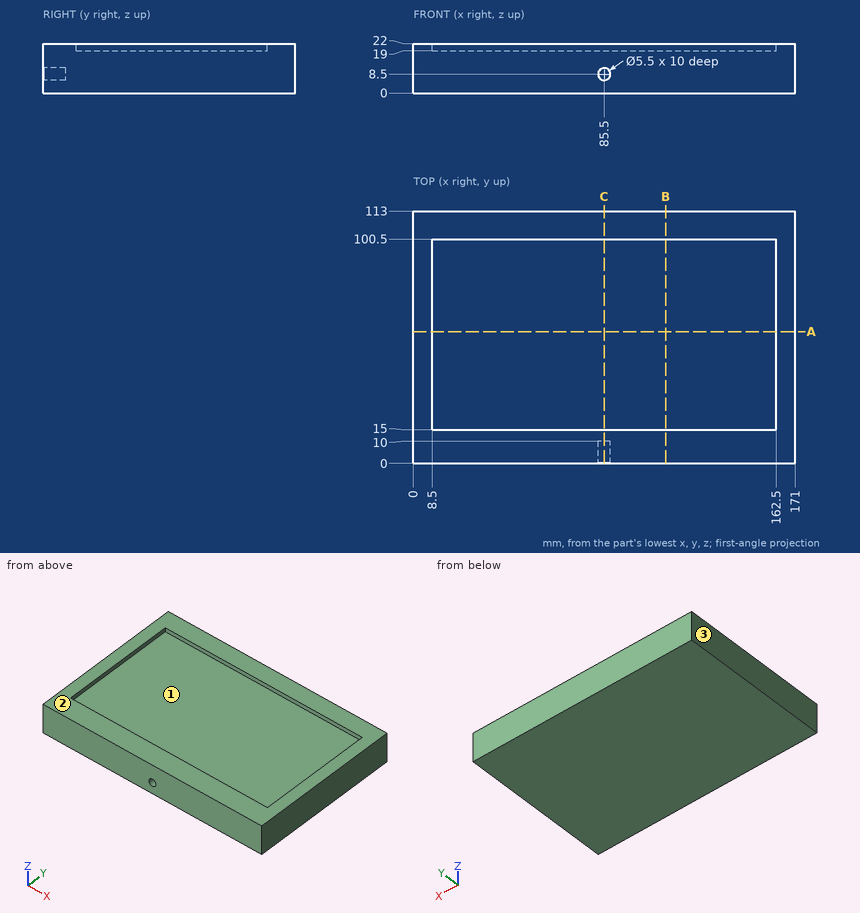
Input: dimensioned drawing with shaded views. Units: mm. Origin: part minimum x, y, z. Give positions to 0.01 mm unless a question says otherwise; leave off trailing zeros. Write each loop counter-clockwise with the first axis right and the second up, starting at its lowest first coordinate (ties: lowest second). Pieces come first, ordered by that corner, then holes. Notation, with made-up numbers: (-32.75, -12) - (-11.75, -12) arc R8 cw to (-11.75, -7) - close; hole circle Ø8 at (49.5, 59.5). An arc over 180 degrees is marked (long way). One line per item, written item: value. Start each with the question number.
Q1. Section query C-C, the plane x = 85.5. Return the cut outline in (y, z), then the cut area to 3 significant figures.
Q2. Draft query along X for the marked faces 1, 2 and 3. Return one class per face: +X half, -X half, draft (parallel to the pull), parting line (faces both ways), or undercut.
Q3. Material intervals for probe 1 along Z at (x, y) = (85.5, 2.75); probe 2 along Y at (x, z) = (102, 21); probe 3 along X at (y, z) = (27.5, 20.5), sorted ascending. Write a range as from..to.
Q4. First-contact query: pin 1 Ø1.6 at (x, z) = (85, 8) entering from -Y; pin 2 Ø10 at (x, y) = (142, 87) entering from +Z; pin 3 Ø8 at (x, y) = (145, 65.5) entering from -Z. Flat tips, straight axial feed; report the tip coordinate or a pass-through.
Q5. Section query B-B, the plane x = 113. Return the cut outline in (y, z), then the cut area to 3 significant figures.
Q6. Section query A-A, the plane y = 59. Return the cut outline in (x, z).
Answer:
1. outline: (0, 0) - (113, 0) - (113, 22) - (100.5, 22) - (100.5, 19) - (15, 19) - (15, 22) - (0, 22) - (0, 11.25) - (10, 11.25) - (10, 5.75) - (0, 5.75) - close
1. area: 2,170 mm2
2. face 1: undercut
2. face 2: draft
2. face 3: -X half
3. probe 1: z = 0..5.75, 11.25..22
3. probe 2: y = 0..15, 100.5..113
3. probe 3: x = 0..8.5, 162.5..171
4. pin 1: stops at y = 10
4. pin 2: stops at z = 19
4. pin 3: stops at z = 0
5. outline: (0, 0) - (113, 0) - (113, 22) - (100.5, 22) - (100.5, 19) - (15, 19) - (15, 22) - (0, 22) - close
5. area: 2,230 mm2
6. outline: (0, 0) - (171, 0) - (171, 22) - (162.5, 22) - (162.5, 19) - (8.5, 19) - (8.5, 22) - (0, 22) - close
